from build123d import *

# Parameters (mm, degrees)
BOSS_EXTRUDE1_DEPTH             = 10
SKETCH2_R                       = 5
CUT_EXTRUDE1_DEPTH              = 11
FILLET1_R                       = 3
CUT_EXTRUDE4_DEPTH              = 11
CUT_EXTRUDE5_DEPTH              = 8
FILLET2_R                       = 3
F_5_0MM_DOWEL_HOLE2_AT_2_COUNT  = 2
F_5_0MM_DOWEL_HOLE2_AT_2_PITCH  = 40
TAP_DRILL_FOR_M5X0_8_TAP1_D     = 4.2
TAP_DRILL_FOR_M5X0_8_TAP1_DEPTH = 2
F_3_0MM_DOWEL_HOLE3_D           = 3
F_5_0MM_DOWEL_HOLE1_D           = 5
F_5_0MM_DOWEL_HOLE1_DEPTH       = 2


with BuildPart() as part:
    # Sketch1 → Boss-Extrude1 (new body)
    with BuildSketch(Plane(origin=(0, 0, 0), x_dir=(1, 0, 0), z_dir=(0, 1, 0))):
        Polygon((0, 88), (0, 8), (8, 0), (88, 0), (96, 8), (96, 88), (88, 96), (8, 96), align=None)
    extrude(amount=BOSS_EXTRUDE1_DEPTH)

    # Sketch2 → Cut-Extrude1 (cut, through all)
    with BuildSketch(Plane(origin=(0, 0, 0), x_dir=(-1, 0, 0), z_dir=(0, -1, 0))):
        with BuildLine():
            Line((-45.411809549, 57.659258263), (-19.071067812, 84))
            Line((-19.071067812, 84), (-76.928932188, 84))
            Line((-76.928932188, 84), (-50.588190451, 57.659258263))
            ThreePointArc((-50.588190451, 57.659258263), (-48, 58), (-45.411809549, 57.659258263))
        make_face()
        with BuildLine():
            Line((-12, 76.928932188), (-38.340741737, 50.588190451))
            ThreePointArc((-38.340741737, 50.588190451), (-38.085551386, 49.305261922), (-38, 48))
            ThreePointArc((-38, 48), (-38.085551386, 46.694738078), (-38.340741737, 45.411809549))
            Line((-38.340741737, 45.411809549), (-12, 19.071067812))
            Line((-12, 19.071067812), (-12, 76.928932188))
        make_face()
        with BuildLine():
            Line((-19.071067812, 12), (-45.411809549, 38.340741737))
            ThreePointArc((-45.411809549, 38.340741737), (-48, 38), (-50.588190451, 38.340741737))
            Line((-50.588190451, 38.340741737), (-76.928932188, 12))
            Line((-76.928932188, 12), (-19.071067812, 12))
        make_face()
        with BuildLine():
            ThreePointArc((-57.659258263, 45.411809549), (-58, 48), (-57.659258263, 50.588190451))
            Line((-57.659258263, 50.588190451), (-84, 76.928932188))
            Line((-84, 76.928932188), (-84, 19.071067812))
            Line((-84, 19.071067812), (-57.659258263, 45.411809549))
        make_face()
        with Locations((-48, 48)):
            Circle(SKETCH2_R)
    extrude(amount=-CUT_EXTRUDE1_DEPTH, mode=Mode.SUBTRACT)

    # Fillet1
    fillet1_edges = [part.edges().sort_by_distance(p)[0] for p in [
        (50.588190451, 5, -38.340741737),
        (45.411809549, 5, -38.340741737),
        (19.071067812, 5, -12),
        (76.928932188, 5, -12),
        (38.340741737, 5, -45.411809549),
        (38.340741737, 5, -50.588190451),
        (12, 5, -76.928932188),
        (12, 5, -19.071067812),
        (57.659258263, 5, -50.588190451),
        (57.659258263, 5, -45.411809549),
        (84, 5, -19.071067812),
        (84, 5, -76.928932188),
        (45.411809549, 5, -57.659258263),
        (50.588190451, 5, -57.659258263),
        (76.928932188, 5, -84),
        (19.071067812, 5, -84),
    ]]
    fillet(fillet1_edges, radius=FILLET1_R)

    # Sketch5 → Cut-Extrude4 (cut, through all)
    with BuildSketch(Plane(origin=(0, 10, 0), x_dir=(1, 0, 0), z_dir=(0, 1, 0))):
        Polygon((8, 0), (8, 20.5), (0, 20.5), (0, 8), align=None)
        Polygon((96, 8), (88, 0), (88, 20.5), (96, 20.5), align=None)
        Polygon((96, 75.5), (88, 75.5), (88, 96), (96, 88), align=None)
        Polygon((8, 96), (8, 75.5), (0, 75.5), (0, 88), align=None)
    extrude(amount=-CUT_EXTRUDE4_DEPTH, mode=Mode.SUBTRACT)

    # Sketch6 → Cut-Extrude5 (cut)
    with BuildSketch(Plane(origin=(0, 10, 0), x_dir=(1, 0, 0), z_dir=(0, 1, 0))):
        Polygon((86, 73.5), (86, 94), (10, 94), (10, 73.5), (2, 73.5), (2, 22.5), (10, 22.5), (10, 2), (86, 2), (86, 22.5), (94, 22.5), (94, 73.5), align=None)
    extrude(amount=-CUT_EXTRUDE5_DEPTH, mode=Mode.SUBTRACT)

    # Fillet2
    fillet2_edges = [part.edges().sort_by_distance(p)[0] for p in [
        (8, 5, -75.5),
        (88, 5, -75.5),
        (88, 5, -20.5),
        (8, 5, -20.5),
        (94, 6, -73.5),
        (94, 6, -22.5),
        (86, 6, -2),
        (10, 6, -2),
        (2, 6, -22.5),
        (2, 6, -73.5),
        (10, 6, -94),
        (86, 6, -94),
    ]]
    fillet(fillet2_edges, radius=FILLET2_R)

    # Sketch13 → Ø5.0mm Dowel Hole2 (revolve, cut)
    with BuildSketch(Plane(origin=(28, 6, 0), x_dir=(0, -1, 0), z_dir=(1, 0, 0))):
        Polygon((0, 0), (0, 9.002151548), (2.5, 7.5), (2.5, 0), align=None)
    f_5_0mm_dowel_hole2 = revolve(axis=Axis((28, 6, 6.35), (0, 0, -1)), mode=Mode.SUBTRACT)

    # Ø5.0mm Dowel Hole2 at 2: Ø5.0mm Dowel Hole2 ×2
    with Locations(*[(i * F_5_0MM_DOWEL_HOLE2_AT_2_PITCH, 0, 0) for i in range(1, F_5_0MM_DOWEL_HOLE2_AT_2_COUNT)]):
        add(f_5_0mm_dowel_hole2, mode=Mode.SUBTRACT)

    # Tap Drill for M5x0.8 Tap1
    with Locations(Plane.ZY):
        with Locations((-68, 6), (-28, 6)):
            Hole(TAP_DRILL_FOR_M5X0_8_TAP1_D / 2, depth=TAP_DRILL_FOR_M5X0_8_TAP1_DEPTH)

    # Mirror1: Ø5.0mm Dowel Hole2 across plane
    add(f_5_0mm_dowel_hole2.mirror(Plane.XY.offset(-48)), mode=Mode.SUBTRACT)

    # Mirror1 copy 1 sketch → Mirror1 copy 1 (revolve, cut)
    with BuildSketch(Plane(origin=(68, 6, -96), x_dir=(0, -1, 0), z_dir=(1, 0, 0))):
        Polygon((0, 0), (0, -9.002151548), (2.5, -7.5), (2.5, 0), align=None)
    revolve(axis=Axis((68, 6, -102.35), (0, 0, -1)), mode=Mode.SUBTRACT)

    # Ø3.0mm Dowel Hole3 (through all)
    with Locations(Plane(origin=(78, 0, -18), x_dir=(0, 0, -1), z_dir=(0, -1, 0))):
        with Locations((0, 0), (60, 0), (60, -60), (0, -60)):
            Hole(F_3_0MM_DOWEL_HOLE3_D / 2)

    # Ø5.0mm Dowel Hole1
    with Locations(Plane(origin=(96, 6, -68), x_dir=(0, 0, 1), z_dir=(1, 0, 0))):
        with Locations((0, 0), (40, 0)):
            Hole(F_5_0MM_DOWEL_HOLE1_D / 2, depth=F_5_0MM_DOWEL_HOLE1_DEPTH)


solid = part.part
Geometry: final body of the model. Coordinates: model frame, mm. A direction names the side the tool comes from. Give positions to 0.01 mm unless a question says otherwise; leave off trailing zeros. Order: outer loops, then holes, each group sorted by start corner. A loop starts at its lowest first (then second) coordinate and runs counter-clockwise, first axis right, second up. Notation, with made-up numbers: (-33, -33.5) -> (-9, -33.5) arc R14 cw to (-9, -29.5) -> close; hole circle Ø9 at (84.5, -24.75). An arc over 180 degrees is marked (long way). Put each result on its own line as item: value.
Q1. Section C-C, the plane z = -28. Return loops of the section in (x, y), then the cut area to 3 significant figures.
Here are the results:
outline: (0, 0) -> (12, 0) -> (12, 2) -> (2, 2) -> (2, 3.9) -> (0, 3.9) -> close; (0, 8.1) -> (2, 8.1) -> (2, 10) -> (0, 10) -> close; (20.93, 0) -> (35.07, 0) -> (35.07, 2) -> (20.93, 2) -> close; (60.93, 0) -> (75.07, 0) -> (75.07, 2) -> (60.93, 2) -> close; (84, 0) -> (96, 0) -> (96, 3.5) -> (94, 3.5) -> (94, 2) -> (84, 2) -> close; (94, 8.5) -> (96, 8.5) -> (96, 10) -> (94, 10) -> close
area: 118 mm^2
Q2. Section B-B, the plane x = 28. Return loops of the section in (y, z), then the cut area to 3 significant figures.
Here are the results:
outline: (0, -96) -> (3.5, -96) -> (3.5, -94) -> (2, -94) -> (2, -84) -> (0, -84) -> close; (0, -75.07) -> (2, -75.07) -> (2, -60.93) -> (0, -60.93) -> close; (0, -35.07) -> (2, -35.07) -> (2, -20.93) -> (0, -20.93) -> close; (0, -12) -> (2, -12) -> (2, -2) -> (3.5, -2) -> (3.5, 0) -> (0, 0) -> close; (8.5, -96) -> (10, -96) -> (10, -94) -> (8.5, -94) -> close; (8.5, -2) -> (10, -2) -> (10, 0) -> (8.5, 0) -> close
area: 117 mm^2
Q3. Pin query (flat end, axial travel): pin 1 (4 mm diameter, centred on y = 6.5, z = -85, fed in from +X); pin 2 (1.5 mm diameter, centred on x = 94, y = 5.5, fed in from -Z); pin 3 (4.5 mm diameter, centred on y = 6, z = -28, fed in from +X). Return the tip coordinate at first contact, or that it passes through.
Here are the results:
pin 1: stops at x = 88
pin 2: stops at z = -75.5
pin 3: stops at x = 2
Q4. Reachability of faces 3 (the face through (88, 5, -9)), 4 (the face through (94, 6, -48)), 5 (the face through (94.986, 5.249, -70.385)), 6 (the face through (72.44, 1.01, -13.81)) from +Z, -Z, +X, -X, +Y, -Y: full face, straight path, thin tool, end or side. Return the list, or none.
Here are the results:
face 3: +Z, +X, +Y, -Y
face 4: +Y
face 5: +X
face 6: +Y, -Y
Q5. Material intervals for L1, parallel to X at y = 6, z = -1.2; L2, parallel to Z at x = 66.5, y = 9; L3, parallel to Y at x = 0.9, z = -28, sorted ascending.
Here are the results:
L1: x = 8 to 25.5, 30.5 to 65.5, 70.5 to 88
L2: z = -96 to -94, -2 to 0
L3: y = 0 to 3.9, 8.1 to 10
Q6. Draft query along Y for faces 1 (the face through (25.89, 4.66, -95.01)), 2 (the face through (10, 6, -14)). Return one class per face: released by +Y, released by -Y, zero draft, split by the parting line, or undercut.
Here are the results:
face 1: undercut
face 2: zero draft
Q7. Section A-A, the plane z = -81. Return loops of the section in (x, y), then the cut area to 3 significant figures.
Here are the results:
outline: (8, 0) -> (23.31, 0) -> (23.31, 2) -> (10, 2) -> (10, 10) -> (8, 10) -> close; (72.69, 0) -> (88, 0) -> (88, 10) -> (86, 10) -> (86, 2) -> (72.69, 2) -> close
area: 93.3 mm^2
Q8. Section D-D, the plane z = -9.5. Return loops of the section in (x, y), then the cut area to 3 significant figures.
Here are the results:
outline: (8, 0) -> (88, 0) -> (88, 10) -> (86, 10) -> (86, 2) -> (10, 2) -> (10, 10) -> (8, 10) -> close
area: 192 mm^2
